Design review of the part built by this model. Coordinates are the model's own, in mm. Face numbers are marked on the shaded views. A direction names the side the tool comes from. Give positions to 0.01 mm unless a question says otherwise; leave off trailing zeros. Order: outer loops, then holes, each group sorted by start corner. A loop starts at its lowest first (then second) coordinate and runs counter-clockwise, first axis right, second up. Notation, with made-up numbers: (44, 25) -> (79, 25) arc R15 ccw to (79, 34) -> close; hole circle Ø9 at (37, 74). An arc over 180 degrees is marked (long way). One line per item, written item: value.
from build123d import *

# Parameters (mm, degrees)
SKETCH1_R           = 6.53
BOSS_EXTRUDE1_DEPTH = 10


with BuildPart() as part:
    # Sketch1 → Boss-Extrude1 (new body)
    with BuildSketch(Plane.XY):
        with BuildLine():
            Line((6.53, -6.941181456), (6.53, -26.94))
            ThreePointArc((6.53, -26.94), (7.408679656, -29.061320344), (9.53, -29.94))
            Line((9.53, -29.94), (24.53, -29.94))
            Line((24.53, -29.94), (24.53, -26.94))
            Line((24.53, -26.94), (12.53, -26.94))
            ThreePointArc((12.53, -26.94), (10.408679656, -26.061320344), (9.53, -23.94))
            Line((9.53, -23.94), (9.53, 0))
            ThreePointArc((9.53, 0), (0, 9.53), (-9.53, 0))
            Line((-9.53, 0), (-9.53, -23.94))
            ThreePointArc((-9.53, -23.94), (-10.408679656, -26.061320344), (-12.53, -26.94))
            Line((-12.53, -26.94), (-24.53, -26.94))
            Line((-24.53, -26.94), (-24.53, -29.94))
            Line((-24.53, -29.94), (-9.53, -29.94))
            ThreePointArc((-9.53, -29.94), (-7.408679656, -29.061320344), (-6.53, -26.94))
            Line((-6.53, -26.94), (-6.53, -6.941181456))
            ThreePointArc((-6.53, -6.941181456), (0, -9.53), (6.53, -6.941181456))
        make_face()
        Circle(SKETCH1_R, mode=Mode.SUBTRACT)
    extrude(amount=BOSS_EXTRUDE1_DEPTH)


solid = part.part
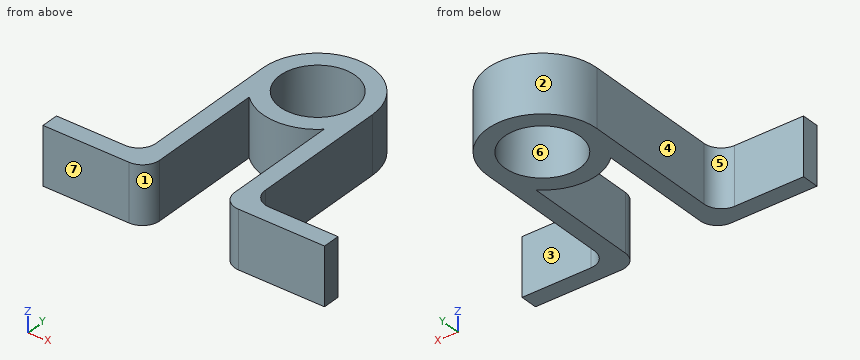
Item 1: Add section D-D on x = -15. Give the boundary of the cut face in (y, z), plus the area to 3 significant figures.
Returned:
outline: (-29.94, 0) -> (-26.94, 0) -> (-26.94, 10) -> (-29.94, 10) -> close
area: 30.0 mm²
Item 2: Draft analysis for pull direction Y (two halves, no side actions). For the marked faces 5, 6 and 7, state which applies: pulls with the +Y half, pulls with the -Y half, needs draft (parallel to the pull), parting line crosses it, or undercut.
Returned:
face 5: pulls with the +Y half
face 6: undercut
face 7: pulls with the -Y half
Item 3: Clearance check with flat-ended pins moving along their axes: P1, Ø3, axis at y = 0.5, z = 7, coming from the -X side; P2, Ø5, axis at y = -19.5, z = 7, coming from the +X side; P3, Ø6, axis at x = 5.5, z = 2, coming from the +Y side. State where each tip first meets the part, or that it passes through.
Returned:
P1: x = -9.53
P2: x = 9.53
P3: y = 9.2
Item 4: Machinability: for the marked faces 1, 2, 3 and 4, which of the approach directions +Z, -Z, +X, -X, +Y, -Y give a long, thin tool a straight path to every point of the face, cutting with its end or side? Answer none if there is none.
Returned:
face 1: +Z, -Z, -Y
face 2: +Z, -Z, +Y
face 3: +Z, -Z, +X, +Y
face 4: +Z, -Z, -X, +Y
Item 5: To check wall thickness, follow line 1 along Y through (x, z) = (0, 7.75); line 2 along X through (y, z) = (5.5, 5.5); line 3 along Y through (x, z) = (-20, 8). State the ranges of each line that lie inside material, in increasing order. Write a range as from..to.
Returned:
line 1: -9.53..-6.53, 6.53..9.53
line 2: -7.78..-3.52, 3.52..7.78
line 3: -29.94..-26.94
Item 6: Add section A-A on y = -17.5. Give the boundary of the cut face in (x, z).
Returned:
outline: (-9.53, 0) -> (-6.53, 0) -> (-6.53, 10) -> (-9.53, 10) -> close; (6.53, 0) -> (9.53, 0) -> (9.53, 10) -> (6.53, 10) -> close
Item 7: Add section C-C on z = 3.25. Give the boundary of the cut face in (x, y), plus the area to 3 significant figures.
Returned:
outline: (-24.53, -29.94) -> (-9.53, -29.94) arc R3 ccw to (-6.53, -26.94) -> (-6.53, -6.94) arc R9.53 ccw to (6.53, -6.94) -> (6.53, -26.94) arc R3 ccw to (9.53, -29.94) -> (24.53, -29.94) -> (24.53, -26.94) -> (12.53, -26.94) arc R3 cw to (9.53, -23.94) -> (9.53, 0) arc R9.53 ccw to (-9.53, 0) -> (-9.53, -23.94) arc R3 cw to (-12.53, -26.94) -> (-24.53, -26.94) -> close; hole circle Ø13.06 at (0, 0)
area: 392 mm²
